Read the model definition and answer for the solid it produces. Units are mm, in the model's axes. Face numbers are marked on the shaded views. A direction names the side the tool comes from. Coordinates: 2 decimals unless noted, no trailing zeros. Write each loop counter-clockwise with the first axis right and the second up, starting at its lowest first coordinate (ties: lowest second). Pieces come first, ordered by that corner, then holes. Notation, with made-up numbers: M 68,59.25 L 107,59.25 A21 ccw 107,64.25 Z; hole C 45,-37.5 d7. An arc over 180 degrees is marked long. Write item = value, one per line.
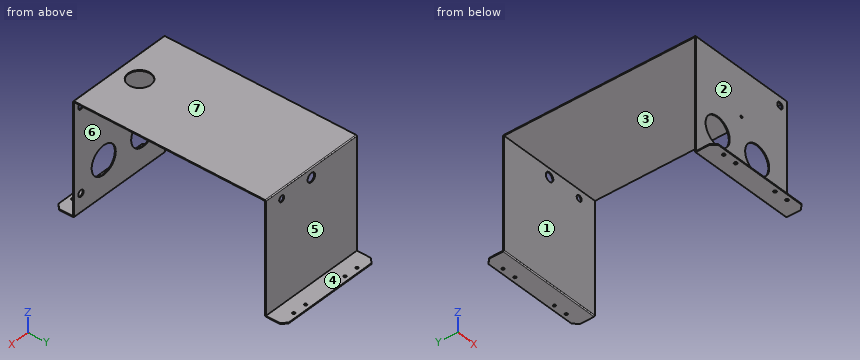
from build123d import *

# Parameters (mm, degrees)
F1_DEPTH  = 230
F3_D      = 48.6
F5_D      = 6.5
F6_D      = 5.5
F7_SIZE   = 10
F9_D      = 61
F9_DEPTH  = 12
F10_D     = 5
F10_DEPTH = 5
F11_D     = 13.72
F11_DEPTH = 5
F13_D     = 12.7
F13_DEPTH = 5
F14_D     = 19.05
F14_DEPTH = 5


with BuildPart() as f1:
    # F0 (on Right) → F1 (new body)
    with BuildSketch(Plane.YZ):
        with BuildLine():
            Line((205, 0), (-205, 0))
            ThreePointArc((-205, 0), (-206.414214, -0.585786), (-207, -2))
            Line((-207, -2), (-207, -238))
            Line((-207, -238), (-247, -238))
            Line((-247, -238), (-247, -240))
            Line((-247, -240), (-207, -240))
            ThreePointArc((-207, -240), (-205.585786, -239.414214), (-205, -238))
            Line((-205, -238), (-205, -2))
            Line((-205, -2), (205, -2))
            Line((205, -2), (205, -238))
            ThreePointArc((205, -238), (205.585786, -239.414214), (207, -240))
            Line((207, -240), (247, -240))
            Line((247, -240), (247, -238))
            Line((247, -238), (207, -238))
            Line((207, -238), (207, -2))
            ThreePointArc((207, -2), (206.414214, -0.585786), (205, 0))
        make_face()
    extrude(amount=F1_DEPTH)

    # F3 (through all)
    with Locations(Plane.XY):
        with Locations((115, -162)):
            Hole(F3_D / 2)

    # F5 (through all)
    with Locations(Plane.XY.offset(-238)):
        with Locations((35, -237), (65, -237), (165, -237), (195, -237)):
            Hole(F5_D / 2)

    # F6 (through all)
    with Locations(Plane.XY.offset(-238)):
        with Locations((35, 237), (65, 237), (165, 237), (195, 237)):
            Hole(F6_D / 2)

    # F7
    f7_edges = [f1.edges().sort_by_distance(p)[0] for p in [
        (0, -247, -239),
        (230, -247, -239),
        (230, 247, -239),
        (0, 247, -239),
    ]]
    chamfer(f7_edges, length=F7_SIZE)

    # F9
    with Locations(Plane.XZ.offset(207)):
        with Locations((55, -165), (155, -165)):
            Hole(F9_D / 2, depth=F9_DEPTH)

    # F10
    with Locations(Plane.XZ.offset(207)):
        with Locations((115, -100)):
            Hole(F10_D / 2, depth=F10_DEPTH)

    # F11
    with Locations(Plane.XZ.offset(207)):
        with Locations((212.5, -20), (212.5, -200)):
            Hole(F11_D / 2, depth=F11_DEPTH)

    # F13
    with Locations(Plane(origin=(0, 207, 0), x_dir=(-1, 0, 0), z_dir=(0, 1, 0))):
        with Locations((-190, -20)):
            Hole(F13_D / 2, depth=F13_DEPTH)

    # F14
    with Locations(Plane(origin=(0, 207, 0), x_dir=(-1, 0, 0), z_dir=(0, 1, 0))):
        with Locations((-115, -20)):
            Hole(F14_D / 2, depth=F14_DEPTH)


solid = f1.part
Item 1: Find section D-D (y = 144). Determine the outline of the cut face in (x, z), and give its area (3 significant figures).
Worked answers:
outline = M 0,-2 L 230,-2 L 230,0 L 0,0 Z
area = 460 mm²
Item 2: Find section B-B (z = -35). Determine the outline of the cut face in (x, y), and give its area (3 significant figures).
Worked answers:
outline = M 0,-207 L 230,-207 L 230,-205 L 0,-205 Z; M 0,205 L 230,205 L 230,207 L 0,207 Z
area = 920 mm²
Item 3: Find section A-A (x = 212.5). Determine the outline of the cut face in (y, z).
Worked answers:
outline = M -247,-240 L -207,-240 A2 ccw -205,-238 L -205,-206.86 L -207,-206.86 L -207,-238 L -247,-238 Z; M -207,-193.14 L -205,-193.14 L -205,-26.86 L -207,-26.86 Z; M -207,-13.14 L -205,-13.14 L -205,-2 L 205,-2 L 205,-238 A2 ccw 207,-240 L 247,-240 L 247,-238 L 207,-238 L 207,-2 A2 ccw 205,0 L -205,0 A2 ccw -207,-2 Z
Item 4: Flat-ended cylindrical pins translate along their axes: pin 1 (6 mm diameter, centred on x = 195.5, z = -109.5, fed in from +Y); pin 2 (6.5 mm diameter, centred on x = 65, y = 237, fed in from +Z); pin 3 (5 mm diameter, centred on x = 36.5, z = -130, fed in from -Y); pin 4 (6 mm diameter, centred on x = 195, y = -237, fed in from +Z). Find the tip coordinate at first contact, or state that the pin passes through.
Worked answers:
pin_1 = 207
pin_2 = -238
pin_3 = -207
pin_4 = through
Item 5: Which of the six approach directions +Z, -Z, +X, -X, +Y, -Y give full straight-line access (tool end or side, diameter ignored) to the marked faces 5, 6 and 7?
Worked answers:
face_5 = +Z, +X, -X, +Y
face_6 = -Z, +X, -X
face_7 = +Z, +X, -X, +Y, -Y
Item 6: Find section C-C (z = -170). Determine the outline of the cut face in (x, y), and give its area (3 significant figures).
Worked answers:
outline = M 0,-207 L 24.91,-207 L 24.91,-205 L 0,-205 Z; M 0,205 L 230,205 L 230,207 L 0,207 Z; M 85.09,-207 L 124.91,-207 L 124.91,-205 L 85.09,-205 Z; M 185.09,-207 L 230,-207 L 230,-205 L 185.09,-205 Z
area = 679 mm²
Item 7: For a pull along Y with two mould halves and no side action, classify the marked faces 1, 2, 3 and 4 as released by +Y, released by -Y, zero draft, split by the parting line, or undercut.
Worked answers:
face_1 = undercut
face_2 = released by -Y
face_3 = undercut
face_4 = zero draft
Item 8: Consider line 1 along X through (y, z) = (-237, -239); line 2 along Y through (x, z) = (12, -145); line 3 along Z through (x, y) = (212.5, -205.55). Determine where each line is inside the solid, lowest interval first. Write a range as from..to.
Worked answers:
line_1 = 0..31.75, 38.25..61.75, 68.25..161.75, 168.25..191.75, 198.25..230
line_2 = -207..-205, 205..207
line_3 = -239.38..-206.86, -193.14..-26.86, -13.14..-0.08
